Design review of the part built by this model. Coordinates are the model's own, in mm. Face numbers are marked on the shaded views. A direction names the side the tool comes from. Coordinates: 2 decimals unless noted, no trailing zeros. Write each loop counter-clockwise with the first axis right and the second up, starting at its lowest first coordinate (ties: lowest second). Pieces come first, ordered by that corner, then holes. Notation, with made-up numbers: (-35, 21) - (4, 21) arc R11 ccw to (4, 39) - close; hole circle Ø9 at (26, 71). An arc over 180 degrees is marked (long way). Use a Markdown table: item, result.
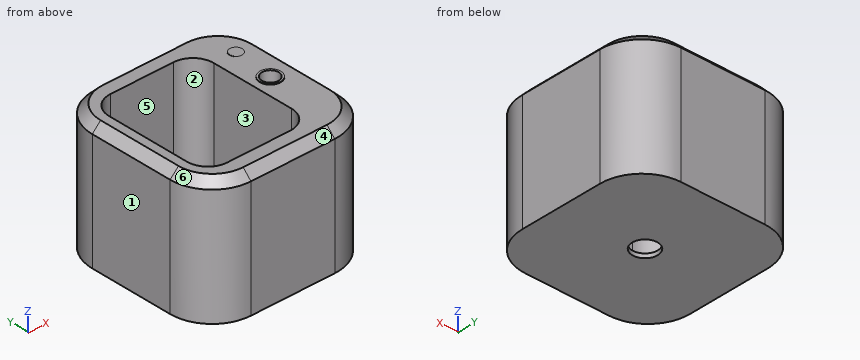
from build123d import *

# Parameters (mm, degrees)
F0_W      = 101.6
F0_H      = 101.6
F1_DEPTH  = 76.2
F3_R      = 25.4
F4_SIZE   = 5.08
F5_DEPTH  = 73.66
F6_R      = 7.676164
F7_DEPTH  = 25.4
F8_R      = 6.35
F9_DEPTH  = 0.254
F10_R     = 5.08
F11_DEPTH = 76.2
F12_R     = 3.81
F13_DEPTH = 0.0254


with BuildPart() as f1:
    # F0 (on Top) → F1 (new body)
    with BuildSketch(Plane.XY):
        Rectangle(F0_W, F0_H)
    extrude(amount=F1_DEPTH)

    # F3
    f3_edges = [f1.edges().sort_by_distance(p)[0] for p in [
        (-50.8, 50.8, 38.1),
        (50.8, 50.8, 38.1),
        (50.8, -50.8, 38.1),
        (-50.8, -50.8, 38.1),
    ]]
    fillet(f3_edges, radius=F3_R)

    # F4
    f4_edges = [f1.edges().sort_by_distance(p)[0] for p in [
        (-50.8, 0, 76.2),
    ]]
    chamfer(f4_edges, length=F4_SIZE)

    # F2 (on face) → F5 (cut)
    with BuildSketch(Plane.XY.offset(76.2)):
        with BuildLine():
            Line((10.16, 38.1), (-27.94, 38.1))
            ThreePointArc((-27.94, 38.1), (-36.920256, 34.380256), (-40.64, 25.4))
            Line((-40.64, 25.4), (-40.64, -25.4))
            ThreePointArc((-40.64, -25.4), (-36.920256, -34.380256), (-27.94, -38.1))
            Line((-27.94, -38.1), (10.16, -38.1))
            ThreePointArc((10.16, -38.1), (19.140256, -34.380256), (22.86, -25.4))
            Line((22.86, -25.4), (22.86, 25.4))
            ThreePointArc((22.86, 25.4), (19.140256, 34.380256), (10.16, 38.1))
        make_face()
    extrude(amount=-F5_DEPTH, mode=Mode.SUBTRACT)

    # F6 (on face) → F7 (cut)
    with BuildSketch(Plane.XY.offset(2.54)):
        Circle(F6_R)
    extrude(amount=-F7_DEPTH, mode=Mode.SUBTRACT)

    # F8 (on face) → F9 (join)
    with BuildSketch(Plane.XY.offset(76.2)):
        with Locations((33.531968, 0)):
            Circle(F8_R)
    extrude(amount=F9_DEPTH)

    # F10 (on face) → F11 (cut)
    with BuildSketch(Plane.XY.offset(76.454)):
        with Locations((33.531968, 0)):
            Circle(F10_R)
    extrude(amount=-F11_DEPTH, mode=Mode.SUBTRACT)

    # F12 (on face) → F13 (join)
    with BuildSketch(Plane.XY.offset(76.2)):
        with Locations((36.258892, 25.4)):
            Circle(F12_R)
    extrude(amount=F13_DEPTH)


solid = f1.part
(1) Take a section at A-A on y = 0. Write out the cut boundary in (x, z), and give its area (3 significant figures).
Determined:
| item | result |
|---|---|
| outline | (-50.8, 0) - (-7.68, 0) - (-7.68, 2.54) - (-40.64, 2.54) - (-40.64, 76.2) - (-45.72, 76.2) - (-50.8, 71.12) - close; (7.68, 0) - (50.8, 0) - (50.8, 71.12) - (45.72, 76.2) - (39.88, 76.2) - (39.88, 76.45) - (38.61, 76.45) - (38.61, 0.25) - (28.45, 0.25) - (28.45, 76.45) - (27.18, 76.45) - (27.18, 76.2) - (22.86, 76.2) - (22.86, 2.54) - (7.68, 2.54) - close |
| area | 2,230 mm2 |
(2) Machinability: for the marked faces 5 and 6, which of the approach directions +Z, -Z, +X, -X, +Y, -Y give a long, thin tool a straight path to every point of the face, cutting with its end or side? Answer none if there is none.
Determined:
| item | result |
|---|---|
| face 5 | +Z |
| face 6 | +Z, -X, -Y |
(3) For pin 1 (2 mm diameter, centred on x = -28.5, z = 32.5, fed in from +Y); pin 2 (3 mm diameter, centred on x = 33, y = 0.5, fed in from +Z); pin 3 (6 mm diameter, centred on x = 36.5, y = 24, fed in from +Z), all flat-tipped, find the tip position at first contact; note any pin that passes through.
Determined:
| item | result |
|---|---|
| pin 1 | y = 50.71 |
| pin 2 | z = 0.25 |
| pin 3 | z = 76.23 |
(4) Take a section at C-C on z = 60.5. Write out the cut boundary in (x, y).
Determined:
| item | result |
|---|---|
| outline | (-50.8, -25.4) arc R25.4 ccw to (-25.4, -50.8) - (25.4, -50.8) arc R25.4 ccw to (50.8, -25.4) - (50.8, 25.4) arc R25.4 ccw to (25.4, 50.8) - (-25.4, 50.8) arc R25.4 ccw to (-50.8, 25.4) - close; hole (-40.64, -25.4) arc R12.7 ccw to (-27.94, -38.1) - (10.16, -38.1) arc R12.7 ccw to (22.86, -25.4) - (22.86, 25.4) arc R12.7 ccw to (10.16, 38.1) - (-27.94, 38.1) arc R12.7 ccw to (-40.64, 25.4) - close; hole circle Ø10.16 at (33.53, 0) |
(5) Take a section at B-B on x = -21. Write out the cut boundary in (y, z), and give its area (3 significant figures).
Determined:
| item | result |
|---|---|
| outline | (-50.8, 0) - (50.8, 0) - (50.8, 71.12) - (45.72, 76.2) - (38.1, 76.2) - (38.1, 2.54) - (-38.1, 2.54) - (-38.1, 76.2) - (-45.72, 76.2) - (-50.8, 71.12) - close |
| area | 2,100 mm2 |
(6) Take a section at D-D on x = 0. Write out the cut boundary in (y, z).
Determined:
| item | result |
|---|---|
| outline | (-50.8, 0) - (-7.68, 0) - (-7.68, 2.54) - (-38.1, 2.54) - (-38.1, 76.2) - (-45.72, 76.2) - (-50.8, 71.12) - close; (7.68, 0) - (50.8, 0) - (50.8, 71.12) - (45.72, 76.2) - (38.1, 76.2) - (38.1, 2.54) - (7.68, 2.54) - close |
(7) For L1, parallel to Y at x = 0, z = 0.8; L2, parallel to X at y = -18, z = 30; L3, parallel to Y at x = -20, z = 58, list the stretches that pass through material, from the lowest coordinate up. Write a range as from..to.
Determined:
| item | result |
|---|---|
| L1 | -50.8..-7.68, 7.68..50.8 |
| L2 | -50.8..-40.64, 22.86..50.8 |
| L3 | -50.8..-38.1, 38.1..50.8 |
(8) Draft analysis for pull direction Y (two halves, no side actions). For the marked faces 1, 2, 3 and 4, state which applies: +Y half, -Y half, draft (parallel to the pull), parting line (faces both ways), or undercut.
Determined:
| item | result |
|---|---|
| face 1 | draft |
| face 2 | undercut |
| face 3 | undercut |
| face 4 | -Y half |
